from build123d import *

# Parameters (mm, degrees)
EXTRUDE1_DEPTH = 38.1
SKETCH2_R      = 7.543563031
SKETCH2_R_2    = 1.586948076
EXTRUDE2_DEPTH = 38.1


with BuildPart() as part:
    # Sketch1 → Extrude1 (new body)
    with BuildSketch(Plane(origin=(0, 0, 0), x_dir=(0, 0, -1), z_dir=(1, 0, 0))):
        with BuildLine():
            Line((34.023739696, 28.939470853), (91.107488572, 28.939470853))
            ThreePointArc((91.107488572, 28.939470853), (93.758821762, 29.562065849), (95.855917312, 31.299702884))
            Line((95.855917312, 31.299702884), (109.047015974, 48.716075337))
            Line((109.047015974, 48.716075337), (103.985043986, 52.54999495))
            Line((103.985043986, 52.54999495), (92.699615676, 37.649702884))
            ThreePointArc((92.699615676, 37.649702884), (90.602520127, 35.912065849), (87.951186937, 35.289470853))
            Line((87.951186937, 35.289470853), (34.023739696, 35.289470853))
            Line((34.023739696, 35.289470853), (34.023739696, 28.939470853))
        make_face()
    extrude(amount=-EXTRUDE1_DEPTH)

    # Sketch2 → Extrude2 (cut)
    with BuildSketch(Plane(origin=(0, 0, 0), x_dir=(1, 0, 0), z_dir=(0, 1, 0))):
        with Locations(Location((-19.05, 61.225007573, 0), (0, 0, 90))):
            Circle(SKETCH2_R)
        with Locations(Location((-32.67765431, 61.225007573, 0), (0, 0, 90))):
            Circle(SKETCH2_R_2)
        with Locations(Location((-19.05, 74.852661883, 0), (0, 0, 90))):
            Circle(SKETCH2_R_2)
        with Locations(Location((-5.42234569, 61.225007573, 0), (0, 0, 90))):
            Circle(SKETCH2_R_2)
        with Locations(Location((-19.05, 47.597353263, 0), (0, 0, 90))):
            Circle(SKETCH2_R_2)
    extrude(amount=EXTRUDE2_DEPTH, mode=Mode.SUBTRACT)


solid = part.part
Check sheet for the modelled part. Datum: model origin and axes. Units: mm. A direction names the side the tool comes from. Give positions to 0.01 mm unless a question says otherwise; leave off trailing zeros. Loops run counter-clockwise (first coordinate to the right, second up) from the corner with the lowest first, then second, coordinate; pieces in that order, holes last. Notation, with made-up numbers: M 4,-17.5 L 22,-17.5 A18 cw 22,-12.5 Z; hole C 57,88 d9. An arc over 180 degrees is marked long. Answer as a JSON object with one key per item and string values. Group by question number.
Q1. Access from +Z, -Z, +X, -X, +Y, -Y to the whole of each face (thin tool, end or side, straight path). Record for faces 1 (the cylindrical face through (-18.442, 32.07, -49.063)), 2 (the flat face through (-10, 35.289, -61)).
Q2. Material ranges on line 1 along Y through (x, z) = (-28, -58); line 2 along Z through (x, y) = (-13, 32.5); line 3 along X through (y, z) = (30, -47), recorded low to high. Write a range as [from, to].
Q3. Cross-section at C-C on y = 51. Record the cut outline in (x, z).
Q4. Go/stop test with flat-tipped pins: P1, Ø2, axis at x = -9, z = -93.5, coming from the -Y side; P2, Ø11.5, axis at x = -27.5, z = -57.5, coming from the +Y side; P3, Ø1.5, axis at y = 37, z = -53.5, coming from the -X side; P4, Ø1.5, axis at x = -5, y = 42, coming from the +Z side. Record where each tip stops, or that it passes through.
Q5. Release check for a two-part mould opening along X. For faces 3 (the cylindrical face through (-18.4, 32.1, -76.3)), 4 (the flat face through (-18.783, 50.606, -106.551)), 5 (the cylindrical face through (-32.75, 32.07, -59.64)), 6 (the flat face through (0, 35, -74)) record: released by +X, released by -X, zero draft, split by the parting line, or undercut.
Q6. Cross-section at B-B on z = -39.5. Record the cut outline in (x, y).
Q7. Cross-section at A-A on x = -19.05. Record the cut outline in (y, z).
Evaluation:
{
 "1": {"face 1": "+Y, -Y", "face 2": "+Z, +X, -X, +Y"},
 "2": {"line 1": "y = [28.94, 35.29]", "line 2": "z = [-96.77, -65.73], [-56.72, -34.02]", "line 3": "x = [-38.1, -20.52], [-17.58, 0]"},
 "3": {"outline": "M -38.1,-106.03 L 0,-106.03 L 0,-102.81 L -38.1,-102.81 Z"},
 "4": {"P1": "stops at y = 29.1", "P2": "stops at y = 35.29", "P3": "passes through", "P4": "stops at z = -95.43"},
 "5": {"face 3": "undercut", "face 4": "zero draft", "face 5": "undercut", "face 6": "released by +X"},
 "6": {"outline": "M -38.1,28.94 L 0,28.94 L 0,35.29 L -38.1,35.29 Z"},
 "7": {"outline": "M 28.94,-91.11 A5.96 ccw 31.3,-95.86 L 48.72,-109.05 L 52.55,-103.99 L 37.65,-92.7 A5.96 cw 35.29,-87.95 L 35.29,-76.44 L 28.94,-76.44 Z; M 28.94,-73.27 L 35.29,-73.27 L 35.29,-68.77 L 28.94,-68.77 Z; M 28.94,-53.68 L 35.29,-53.68 L 35.29,-49.18 L 28.94,-49.18 Z; M 28.94,-46.01 L 35.29,-46.01 L 35.29,-34.02 L 28.94,-34.02 Z"}
}
